Drawing for the job (mm, zero at the part's lowest x, y, z). Round coordinates to 2 decimals unless told otherwise and drop trailing zeros. Order: outer loops, then holes, each group sorted by start corner. A loop starts at its lowest first (then second) coordinate and runs counter-clockwise, first axis right, second up. Notation, with made-up numbers: (72, 13.25) - (115, 13.25) arc R28 ccw to (115, 46.25) - close; hole circle Ø4 at (76.5, 31). An arc over 180 degrees is marked (long way). Put each result on its own line as item: value. Start each with the question number.
Item 1: Probe probe 1 along X at (y, z) = (6, 1.25) (1 decimal); probe 2 along X at (y, z) = (43.5, 1) (1 decimal); probe 3 along Y at (x, z) = (9.5, 4.5) (1 decimal). List the from-to ranges inside material, lowest first.
Item 2: Saw through at B-B on y = 4.5. State how many separate pieces and enclosed holes the cut face has, plus the area to 3 significant figures.
Item 3: Pin check, flat tips, straight feed: pin 1 Ø3 at (y, z) = (4.5, 4.5) entering from +X (1 decimal); pin 2 Ø2 at (y, z) = (11.5, 4.5) entering from -X (1 decimal); pin 3 Ø1.9 at (x, z) = (107.5, 4.5) entering from +Y (1 decimal). Stop position of each tip, or through.
Item 4: Saw through at A-A on x = 9. List the corners of the cut face in (y, z), plus the area to 3 significant figures.
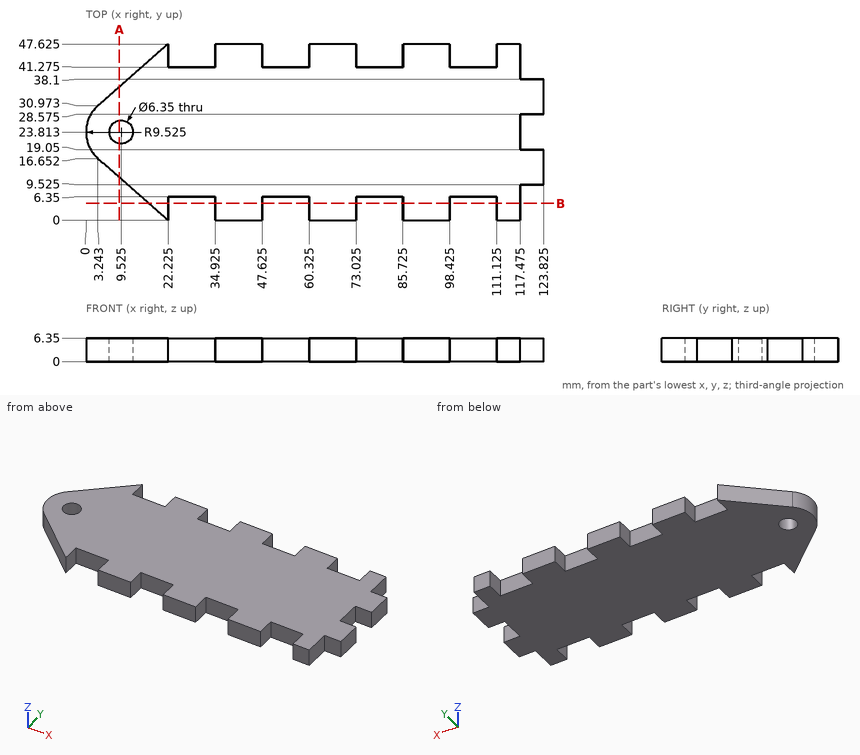
Results found:
1. probe 1: x = 15.4 to 22.2, 34.9 to 47.6, 60.3 to 73, 85.7 to 98.4, 111.1 to 117.5
1. probe 2: x = 17.5 to 22.2, 34.9 to 47.6, 60.3 to 73, 85.7 to 98.4, 111.1 to 117.5
1. probe 3: y = 11.2 to 20.6, 27 to 36.5
2. separate pieces: 5
2. enclosed holes: 0
2. area: 315 mm²
3. pin 1: stops at x = 117.5
3. pin 2: stops at x = 8
3. pin 3: stops at y = 41.3
4. outline: (11.6, 0) - (20.68, 0) - (20.68, 6.35) - (11.6, 6.35) - close; (26.94, 0) - (36.02, 0) - (36.02, 6.35) - (26.94, 6.35) - close
4. area: 115 mm²
